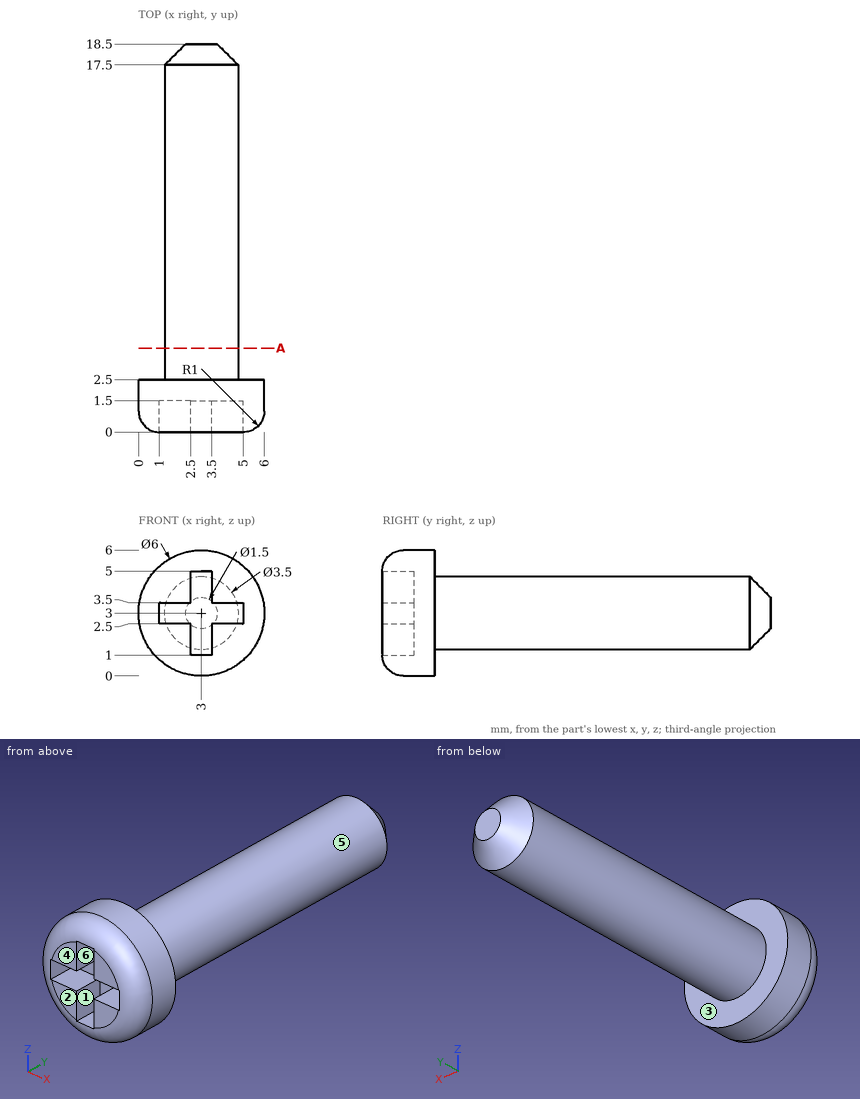
For this review, use the dimensioned drawing (mm, ordinates from the lowest corner) and the shaded views. A direction names the side the tool comes from. Coordinates: 2 decimals unless noted, no trailing zeros. Write each loop counter-clockwise with the first axis right and the second up, starting at its lowest first coordinate (ties: lowest second). Pieces come first, ordered by that corner, then holes. Notation, with made-up numbers: (17.25, -37) -> (48.25, -37) arc R23 ccw to (48.25, -18) -> close; hole circle Ø10 at (43, -26.5). An arc over 180 degrees is marked (long way). Write each question's results on one line, items separated by ' | '. Start each with the question number.
(1) Tool access review of the marked faces 1, 2 and 3: name each direction out of +Z, -Z, +X, -X, +Y, -Y from which nothing blocks a thin tool from reaching the whole face with its end or side.
(2) Clearance check with flat-ended pins moving along their axes: P1, Ø0.5, axis at x = 4.5, y = 0.5, coming from the -Z side; P2, Ø1.5, axis at x = 1, y = 12.5, coming from the -Z side; P3, Ø1.2, axis at y = 0.5, z = 1.5, coming from the -X side. State where each tip first meets the part, or that it passes through.
(3) The part is to be moulded in two halves that separate along X. For the marked faces 4, 5 and 6, say which applies: pulls with the +X half, pulls with the -X half, needs draft (parallel to the pull), parting line crosses it, or undercut.
(4) Take a section at A-A on y = 4. Write out the cut boundary in (x, z), and give its area (3 significant figures).
(5) For line 1 along Y through (x, z) = (4, 4.5); line 2 along X through (y, z) = (14.25, 3.75); line 3 along Z through (x, y) = (3.5, 10.25), list the stretches that pass through material, from the lowest coordinate up. Write a range as from..to.
Results found:
1) face 1: -Y | face 2: +Z, -Z, +X, -X, -Y | face 3: +Y
2) P1: stops at z = 0.37 | P2: stops at z = 1.78 | P3: stops at x = 0.19
3) face 4: needs draft | face 5: parting line crosses it | face 6: undercut
4) outline: circle Ø3.5 at (3, 3) | area: 9.62 mm2
5) line 1: y = 0..2.5 | line 2: x = 1.42..4.58 | line 3: z = 1.32..4.68
